Input: part model. Units: mm. Frame: model coordinates. Face numbers are marked on the shaded views. A direction names the side the tool comes from. Coordinates: 2 decimals unless noted, no trailing zeros. Loops run counter-clockwise (first coordinate to the right, second up) from the corner with the lowest first, then second, coordinate; pieces in that order, holes last.
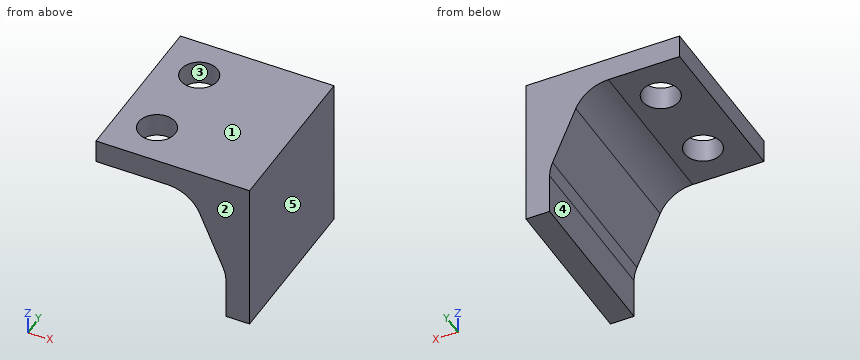
```python
from build123d import *

# Parameters (mm, degrees)
BOSS_EXTRUDE1_DEPTH = 7
CUT_EXTRUDE1_REACH  = 20.412
SKETCH3_R           = 1.55


with BuildPart() as part:
    # Sketch1 → Boss-Extrude1 (new body)
    with BuildSketch(Plane(origin=(0, 0, 0), x_dir=(1, 0, 0), z_dir=(0, 1, 0))):
        with BuildLine():
            Line((0, 0), (-13, 0))
            Line((-13, 0), (-13, 2))
            Line((-13, 2), (-6.966770758, 2))
            ThreePointArc((-6.966770758, 2), (-5.321958583, 2.49109727), (-4.215654921, 3.803604727))
            Line((-4.215654921, 3.803604727), (-2.248884163, 8.326202151))
            ThreePointArc((-2.248884163, 8.326202151), (-2.062880024, 8.911593133), (-2, 9.522597424))
            Line((-2, 9.522597424), (-2, 13))
            Line((-2, 13), (0, 13))
            Line((0, 13), (0, 0))
        make_face()
    extrude(amount=BOSS_EXTRUDE1_DEPTH)

    # Sketch3 → Cut-Extrude1 (cut, up to next)
    with BuildSketch(Plane(origin=(0, 0, -2), x_dir=(-1, 0, 0), z_dir=(0, 0, -1)), mode=Mode.PRIVATE) as cut_extrude1_sk1:
        with Locations((9.621320344, 3.5)):
            Circle(SKETCH3_R)
    cut_extrude1_tool1 = extrude(cut_extrude1_sk1.sketch, amount=-CUT_EXTRUDE1_REACH, mode=Mode.PRIVATE) & part.part
    add(cut_extrude1_tool1.solids().sort_by_distance((-9.62132, 3.5, -2))[0], mode=Mode.SUBTRACT)

    # Mirror1: part across plane


with BuildPart() as part_1:
    add(part.part)
    add(part.part.mirror(Plane(origin=(-6.966770758, 7, -5), x_dir=(0, 0, 1), z_dir=(0, -1, 0))))


solid = part_1.part
```
Item 1: Section query D-D (x = -6). Output: boundary loops of the cut face in (y, z).
Result:
outline: (0, -2.16) - (14, -2.16) - (14, 0) - (0, 0) - close
Item 2: Section query C-C (y = 5.75). Output: boundary loops of the cut face in (x, z).
Result:
outline: (-13, -2) - (-6.97, -2) arc R3 cw to (-4.22, -3.8) - (-2.25, -8.33) arc R3 cw to (-2, -9.52) - (-2, -13) - (0, -13) - (0, 0) - (-13, 0) - close
Item 3: Section query B-B (x = -8.75). Output: boundary loops of the cut face in (y, z).
Result:
outline: (0, -2) - (2.22, -2) - (2.22, 0) - (0, 0) - close; (4.78, -2) - (9.22, -2) - (9.22, 0) - (4.78, 0) - close; (11.78, -2) - (14, -2) - (14, 0) - (11.78, 0) - close
Item 4: Contact query for flat-ended pins moving along their axis: P1, Ø3, axis at y = 6.5, z = -10, coming from the +X side; P2, Ø4, axis at y = 8.5, z = -11, coming from the -X side; P3, Ø4, axis at x = -9.62, y = 3.5, coming from the -Z side. Output: stop coordinate, or through.
Result:
P1: stops at x = 0
P2: stops at x = -2.05
P3: stops at z = -2
Item 5: Reachability of the marked faces 4 and 5 from +Z, -Z, +X, -X, +Y, -Y: full face, straight path, thin tool, end or side. Return the list, or none.
Result:
face 4: -Z, -X, +Y, -Y
face 5: +Z, -Z, +X, +Y, -Y
Item 6: Mould query, pull axis Y, two halves, no side actions, for the marked faces 1, 2 and 3. Classes: +Y half, -Y half, draft (parallel to the pull), parting line (faces both ways), or undercut.
Result:
face 1: draft
face 2: -Y half
face 3: undercut
Item 7: Line query: L1, parallel to Z at x = -11.25, y = 6.75; L2, parallel to X at y = 10.5, z = -1.45. Output: solid intervals per line, ascending.
Result:
L1: z = -2 to 0
L2: x = -13 to -11.17, -8.07 to 0
Item 8: Section query A-A (y = 10.5). Output: boundary loops of the cut face in (x, z), then the cut area to 3 significant figures.
Result:
outline: (-13, -2) - (-11.17, -2) - (-11.17, 0) - (-13, 0) - close; (-8.07, -2) - (-6.97, -2) arc R3 cw to (-4.22, -3.8) - (-2.25, -8.33) arc R3 cw to (-2, -9.52) - (-2, -13) - (0, -13) - (0, 0) - (-8.07, 0) - close
area: 52.9 mm2
